```python
from build123d import *

# Parameters (mm, degrees)
SKETCH1_W           = 42
SKETCH1_H           = 42
BOSS_EXTRUDE1_DEPTH = 10
SKETCH2_W           = 40
SKETCH2_H           = 40
BOSS_EXTRUDE2_DEPTH = 20
SKETCH3_W           = 42
SKETCH3_H           = 42
BOSS_EXTRUDE3_DEPTH = 10
SKETCH4_R           = 11.25
BOSS_EXTRUDE4_DEPTH = 1
CHAMFER1_SIZE       = 4
SKETCH5_R           = 2.5
BOSS_EXTRUDE5_DEPTH = 20
SKETCH6_R           = 1.5
CUT_EXTRUDE1_DEPTH  = 40


with BuildPart() as part:
    # Sketch1 → Boss-Extrude1 (new body)
    with BuildSketch(Plane.XY):
        Rectangle(SKETCH1_W, SKETCH1_H)
    extrude(amount=BOSS_EXTRUDE1_DEPTH)

    # Sketch2 → Boss-Extrude2 (add)
    with BuildSketch(Plane.XY.offset(10)):
        Rectangle(SKETCH2_W, SKETCH2_H)
    extrude(amount=BOSS_EXTRUDE2_DEPTH)

    # Sketch3 → Boss-Extrude3 (add)
    with BuildSketch(Plane.XY.offset(30)):
        Rectangle(SKETCH3_W, SKETCH3_H)
    extrude(amount=BOSS_EXTRUDE3_DEPTH)

    # Sketch4 → Boss-Extrude4 (add)
    with BuildSketch(Plane.XY.offset(40)):
        Circle(SKETCH4_R)
    extrude(amount=BOSS_EXTRUDE4_DEPTH)

    # Chamfer1
    chamfer1_edges = [part.edges().sort_by_distance(p)[0] for p in [
        (20, -20, 20),
        (20, 20, 20),
        (-20, 20, 20),
        (-20, -20, 20),
        (21, -21, 35),
        (21, 21, 35),
        (-21, 21, 35),
        (-21, -21, 35),
        (21, -21, 5),
        (-21, -21, 5),
        (-21, 21, 5),
        (21, 21, 5),
    ]]
    chamfer(chamfer1_edges, length=CHAMFER1_SIZE)

    # Sketch5 → Boss-Extrude5 (add)
    with BuildSketch(Plane.XY.offset(41)):
        Circle(SKETCH5_R)
    extrude(amount=BOSS_EXTRUDE5_DEPTH)

    # Sketch6 → Cut-Extrude1 (cut)
    with BuildSketch(Plane.XY.offset(40)):
        with Locations((-15.5, -15.5)):
            Circle(SKETCH6_R)
        with Locations((-15.5, 15.5)):
            Circle(SKETCH6_R)
        with Locations((15.5, 15.5)):
            Circle(SKETCH6_R)
        with Locations((15.5, -15.5)):
            Circle(SKETCH6_R)
    extrude(amount=-CUT_EXTRUDE1_DEPTH, mode=Mode.SUBTRACT)


solid = part.part
```
Input: part model. Units: mm. Frame: model coordinates. A direction names the side the tool comes from. Round coordinates to 2 decimals unless told otherwise and drop trailing zeros. Order: outer loops, then holes, each group sorted by start corner. A loop starts at its lowest first (then second) coordinate and runs counter-clockwise, first axis right, second up. Notation, with made-up numbers: (80.5, 20) - (123.5, 20) arc R17 cw to (123.5, 47) - close; hole circle Ø2 at (4, 24). An arc over 180 degrees is marked (long way). Answer in a Markdown table with one row per item.
Item 1: Line query: line 1 (Y direction, x = 15.5, z = 16.5); line 2 (Y direction, x = 15.5, z = 30.5); line 3 (X direction, y = 16, z = 16). Output: solid intervals per line, ascending.
Model answer:
| item | result |
|---|---|
| line 1 | y = -20 to -17, -14 to 14, 17 to 20 |
| line 2 | y = -21 to -17, -14 to 14, 17 to 21 |
| line 3 | x = -20 to -16.91, -14.09 to 14.09, 16.91 to 20 |
Item 2: Section query A-A (z = 20.5). Return the cut outline in (x, y).
Model answer:
| item | result |
|---|---|
| outline | (-20, -16) - (-16, -20) - (16, -20) - (20, -16) - (20, 16) - (16, 20) - (-16, 20) - (-20, 16) - close; hole circle Ø3 at (-15.5, -15.5); hole circle Ø3 at (-15.5, 15.5); hole circle Ø3 at (15.5, -15.5); hole circle Ø3 at (15.5, 15.5) |
Item 3: Section query B-B (y = 13). Return the cut outline in (x, z).
Model answer:
| item | result |
|---|---|
| outline | (-21, 0) - (21, 0) - (21, 10) - (20, 10) - (20, 30) - (21, 30) - (21, 40) - (-21, 40) - (-21, 30) - (-20, 30) - (-20, 10) - (-21, 10) - close |
Item 4: Section query D-D (z = 34.5). Return the cut outline in (x, y).
Model answer:
| item | result |
|---|---|
| outline | (-21, -17) - (-17, -21) - (17, -21) - (21, -17) - (21, 17) - (17, 21) - (-17, 21) - (-21, 17) - close; hole circle Ø3 at (-15.5, -15.5); hole circle Ø3 at (-15.5, 15.5); hole circle Ø3 at (15.5, -15.5); hole circle Ø3 at (15.5, 15.5) |
Item 5: Mould query, pull axis Z, two halves, no side actions, for faces 1 (the flat face through (18, 18, 20)), 2 (the flat face through (0, -21, 35)), 3 (the flat face through (-10, 10, 40)). Classes: released by +Z, released by -Z, zero draft, split by the parting line, or undercut.
Model answer:
| item | result |
|---|---|
| face 1 | undercut |
| face 2 | zero draft |
| face 3 | released by +Z |
Item 6: Reachability of faces 4 (the cylindrical face through (-0.54, -2.44, 50.86)), 5 (the flat face through (18, -18, 20)), 6 (the flat face through (-0.1, 20.3, 10)) from +Z, -Z, +X, -X, +Y, -Y: full face, straight path, thin tool, end or side. Return the list, or none.
Model answer:
| item | result |
|---|---|
| face 4 | +Z |
| face 5 | +X, -Y |
| face 6 | none |
Item 7: Section query C-C (x = -18). Return the cut outline in (y, z), then the cut area to 3 significant figures.
Model answer:
| item | result |
|---|---|
| outline | (-20, 0) - (20, 0) - (20, 10) - (18, 10) - (18, 30) - (20, 30) - (20, 40) - (-20, 40) - (-20, 30) - (-18, 30) - (-18, 10) - (-20, 10) - close |
| area | 1,520 mm² |
Item 8: Pin query (flat end, axial travel): pin 1 (1 mm diameter, centred on x = 4, z = 15, fed in from -Y); pin 2 (3.5 mm diameter, centred on x = -15.5, y = -15.5, fed in from +Z); pin 3 (6 mm diameter, centred on y = -2.5, z = 17, fed in from +X). Return the tip coordinate at first contact, or that it passes through.
Model answer:
| item | result |
|---|---|
| pin 1 | stops at y = -20 |
| pin 2 | stops at z = 40 |
| pin 3 | stops at x = 20 |
